Check sheet for the modelled part. Datum: model origin and axes. Units: mm. Face numbers are marked on the shaded views. A direction names the side the tool comes from. Round coordinates to 2 decimals unless told otherwise and drop trailing zeros. Loops run counter-clockwise (first coordinate to the right, second up) from the corner with the lowest first, then second, coordinate; pieces in that order, holes last. Notation, with made-up numbers: (45.25, -1) -> (101.25, -1) arc R13 ccw to (101.25, 20) -> close; hole circle Ø10 at (60.25, -17.75). An arc over 180 degrees is marked (long way). Use one line per item in the form item = value. Start each with the question number.
(1) Sectioned sample at A-A (z = 6). Record the cut outline in (x, y).
(2) Sectioned sample at D-D (x = -27.5). Record the cut outline in (y, z), and give its area (3 significant figures).
(3) Sectioned sample at C-C (y = 13.5). Record the cut outline in (x, z).
(4) Material ranges on probe 1 along X at (y, z) = (11, 19.5); probe 2 along X at (y, z) = (15.25, 4.5); probe 3 along X at (y, z) = (17.5, 40), recorded low to high. Write a range as [from, to].
(5) Set-up check for the marked faces 1, 2, 3 and 4: record each of +Z, -Z, +X, -X, +Y, -Y from which the full face is reachable in a straight line by a thin tool's end or side.
(6) Sectioned sample at B-B (z = 25). Record the cut outline in (x, y), and give its area (3 significant figures).
(7) Go/stop test with flat-tipped pins: pin 1 (4.5 mm diameter, centred on x = 47.52, z = 6, fed in from +Y); pin 2 (1.8 mm diameter, centred on x = 3.37, z = 9.5, fed in from -Y); pin 3 (4 mm diameter, centred on x = -10.5, z = 35, fed in from -Y); pin 4 (4 mm diameter, centred on y = 15, z = 40.5, fed in from -X). Record where each tip stops, or that it passes through.
from build123d import *

# Parameters (mm, degrees)
ESTRUSIONE_ESTRUSIONE1_DEPTH = 50
SCHIZZO2_R                   = 2
TAGLIO_ESTRUSIONE1_DEPTH     = 92.821204916
SCHIZZO3_W                   = 18
SCHIZZO3_H                   = 9
TAGLIO_ESTRUSIONE2_DEPTH     = 35
SCHIZZO4_R                   = 4
SCHIZZO4_R_2                 = 1.5
TAGLIO_ESTRUSIONE3_DEPTH     = 93.4993712
SCHIZZO5_W                   = 129.55
SCHIZZO5_H                   = 1
TAGLIO_ESTRUSIONE4_DEPTH     = 94.767096332


with BuildPart() as part:
    # Schizzo1 → Estrusione-Estrusione1 (new body)
    with BuildSketch(Plane.XY):
        with BuildLine():
            Line((-41.361860063, 6.474046711), (18.188139937, 6.474046711))
            ThreePointArc((18.188139937, 6.474046711), (28.188139937, 16.474046711), (38.188139937, 6.474046711))
            Line((38.188139937, 6.474046711), (53.188139937, 6.474046711))
            Line((53.188139937, 6.474046711), (53.188139937, 11.474046711))
            Line((53.188139937, 11.474046711), (41.848393975, 11.474046711))
            ThreePointArc((41.848393975, 11.474046711), (37.956863927, 18.625242568), (30.330074087, 21.474046711))
            Line((30.330074087, 21.474046711), (-54.59096633, 21.474046711))
            ThreePointArc((-54.59096633, 21.474046711), (-61.816076084, 18.57022327), (-65.022114101, 11.474046711))
            Line((-65.022114101, 11.474046711), (-76.361860063, 11.474046711))
            Line((-76.361860063, 11.474046711), (-76.361860063, 6.474046711))
            Line((-76.361860063, 6.474046711), (-61.361860063, 6.474046711))
            ThreePointArc((-61.361860063, 6.474046711), (-51.361860063, 16.474046711), (-41.361860063, 6.474046711))
        make_face()
    extrude(amount=ESTRUSIONE_ESTRUSIONE1_DEPTH)

    # Schizzo2 → Taglio-Estrusione1 (cut, through all)
    with BuildSketch(Plane(origin=(0, 11.474046711, 0), x_dir=(1, 0, 0), z_dir=(0, 1, 0))):
        with Locations(Location((-70.691860063, -6, 0), (0, 0, 180))):
            Circle(SCHIZZO2_R)
        with Locations(Location((-70.691860063, -44, 0), (0, 0, 180))):
            Circle(SCHIZZO2_R)
        with Locations(Location((47.518139937, -6, 0), (0, 0, 180))):
            Circle(SCHIZZO2_R)
        with Locations(Location((47.518139937, -44, 0), (0, 0, 180))):
            Circle(SCHIZZO2_R)
    extrude(amount=-TAGLIO_ESTRUSIONE1_DEPTH, mode=Mode.SUBTRACT)

    # Schizzo3 → Taglio-Estrusione2 (cut)
    with BuildSketch(Plane.XY.offset(50)):
        with Locations((-11.586860063, 10.974046711)):
            Rectangle(SCHIZZO3_W, SCHIZZO3_H)
    extrude(amount=-TAGLIO_ESTRUSIONE2_DEPTH, mode=Mode.SUBTRACT)

    # Schizzo4 → Taglio-Estrusione3 (cut, through all)
    with BuildSketch(Plane(origin=(0, 21.474046711, 0), x_dir=(1, 0, 0), z_dir=(0, 1, 0))):
        with Locations(Location((-12.130446122, -25, 0), (0, 0, 180))):
            Circle(SCHIZZO4_R)
        with Locations(Location((-27.630446122, -9.5, 0), (0, 0, 180))):
            Circle(SCHIZZO4_R_2)
        with Locations(Location((3.369553878, -9.5, 0), (0, 0, 180))):
            Circle(SCHIZZO4_R_2)
        with Locations(Location((3.369553878, -40.5, 0), (0, 0, 180))):
            Circle(SCHIZZO4_R_2)
        with Locations(Location((-27.630446122, -40.5, 0), (0, 0, 180))):
            Circle(SCHIZZO4_R_2)
    extrude(amount=-TAGLIO_ESTRUSIONE3_DEPTH, mode=Mode.SUBTRACT)

    # Schizzo5 → Taglio-Estrusione4 (cut, through all)
    with BuildSketch(Plane.XY.offset(50)):
        with Locations((-11.586860063, 6.974046711)):
            Rectangle(SCHIZZO5_W, SCHIZZO5_H)
    extrude(amount=-TAGLIO_ESTRUSIONE4_DEPTH, mode=Mode.SUBTRACT)


solid = part.part
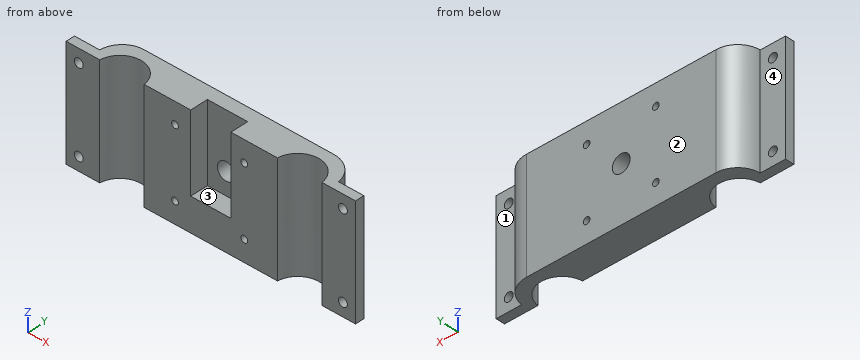
Checks:
q1.outline = (-76.36, 7.47) -> (-72.69, 7.47) -> (-72.69, 11.47) -> (-76.36, 11.47) -> close; (-68.69, 7.47) -> (-61.31, 7.47) arc R10 cw to (-41.41, 7.47) -> (18.24, 7.47) arc R10 cw to (38.14, 7.47) -> (45.52, 7.47) -> (45.52, 11.47) -> (41.85, 11.47) arc R11.63 ccw to (30.33, 21.47) -> (-54.59, 21.47) arc R10.44 ccw to (-65.02, 11.47) -> (-68.69, 11.47) -> close; (49.52, 7.47) -> (53.19, 7.47) -> (53.19, 11.47) -> (49.52, 11.47) -> close
q2.outline = (7.47, 0) -> (21.47, 0) -> (21.47, 8.01) -> (7.47, 8.01) -> close; (7.47, 10.99) -> (21.47, 10.99) -> (21.47, 39.01) -> (7.47, 39.01) -> close; (7.47, 41.99) -> (21.47, 41.99) -> (21.47, 50) -> (7.47, 50) -> close
q2.area = 616 mm2
q3.outline = (-64.74, 0) -> (-58.48, 0) -> (-58.48, 50) -> (-64.74, 50) -> close; (-44.25, 0) -> (21.07, 0) -> (21.07, 50) -> (-2.59, 50) -> (-2.59, 15) -> (-20.59, 15) -> (-20.59, 50) -> (-44.25, 50) -> close; (35.3, 0) -> (41.37, 0) -> (41.37, 50) -> (35.3, 50) -> close; hole circle Ø3 at (-27.63, 9.5); hole circle Ø3 at (-27.63, 40.5); hole circle Ø3 at (3.37, 9.5); hole circle Ø3 at (3.37, 40.5)
q4.probe_1 = [-76.36, -60.28], [-42.44, -20.59], [-2.59, 19.27], [37.11, 53.19]
q4.probe_2 = [-64.14, -56.16], [-46.57, 23.39], [32.98, 40.63]
q4.probe_3 = [-62.79, -29.04], [-26.22, 1.96], [4.78, 39.09]
q5.face_1 = +Z, -Z, +X, +Y
q5.face_2 = +Z, -Z, +X, -X, +Y
q5.face_3 = +Z, -Y
q5.face_4 = +Z, -Z, -X, +Y
q6.outline = (-76.36, 7.47) -> (-61.31, 7.47) arc R10 cw to (-41.41, 7.47) -> (-20.59, 7.47) -> (-20.59, 15.47) -> (-16.13, 15.47) -> (-16.13, 21.47) -> (-54.59, 21.47) arc R10.44 ccw to (-65.02, 11.47) -> (-76.36, 11.47) -> close; (-8.13, 15.47) -> (-2.59, 15.47) -> (-2.59, 7.47) -> (18.24, 7.47) arc R10 cw to (38.14, 7.47) -> (53.19, 7.47) -> (53.19, 11.47) -> (41.85, 11.47) arc R11.63 ccw to (30.33, 21.47) -> (-8.13, 21.47) -> close
q6.area = 1,070 mm2
q7.pin_1 = 11.47
q7.pin_2 = through
q7.pin_3 = 15.47
q7.pin_4 = -64.84
